Autodesk Inventor part; units mm, degrees
ref_plane "YZ Plane" through (0, 0, 0) normal (1, 0, 0) x (0, 1, 0)
ref_plane "XZ Plane" through (0, 0, 0) normal (0, 1, 0) x (-1, 0, 0)
ref_plane "XY Plane" through (0, 0, 0) normal (0, 0, 1) x (1, 0, 0)
sketch "Sketch1" plane through (0, 0, 0) normal (0, 1, 0) x (-1, 0, 0)
  line L0 (33.5, 64.5) -> (-33.5, 64.5)
  line L1 (-33.5, 64.5) -> (-33.5, -64.5)
  line L2 (-33.5, -64.5) -> (33.5, -64.5)
  line L3 (33.5, -64.5) -> (33.5, 64.5)
  line L4 (33.5, 64.5) -> (-33.5, -64.5) construction
  line L5 (-33.5, 64.5) -> (33.5, -64.5) construction
  point P0 (0, 0)
  dimension "d0" = 67
  dimension "d1" = 129
extrude "Extrusion1" add sketch "Sketch1" along normal blind 41
sketch "Sketch2" plane through (-33.5, 0, 64.5) normal (0, 0, 1) x (1, 0, 0)
  circle A0 centre (33.5, 20.5) radius 20.5
  circle A1 centre (33.5, 20.5) radius 18
  point P0 (33.5, 0)
  dimension "d4" = 41
  dimension "d5" = 36
extrude "Extrusion2" add sketch "Sketch2" along normal blind 54 contours A1
extrude "Extrusion3" add sketch "Sketch2" along normal blind 15
sketch "Sketch4" plane through (33.5, 0, -64.5) normal (0, 0, -1) x (-1, 0, 0)
  circle A0 centre (42, 20.5) radius 12.5
  line L0 (67, 0) -> (67, 41)
  point P0 (33.5, 0)
  dimension "d13" = 25
  dimension "d14" = 25
extrude "Extrusion5" add sketch "Sketch4" along normal blind 80
sketch "Sketch5" plane through (0, 0, 0) normal (0, -1, 0) x (1, 0, 0)
  circle A0 centre (0, 51.5) radius 2.5
  circle A1 centre (0, 8.5) radius 2.5
  circle A2 centre (0, -21.5) radius 2
  circle A3 centre (0, -33.5) radius 2.5
  line L0 (-2, 39.5) -> (-2, 37.5)
  line L1 (2, 37.5) -> (2, 39.5)
  arc A4 (2, 39.5) -> (-2, 39.5) centre (0, 39.5) ccw
  arc A5 (-2, 37.5) -> (2, 37.5) centre (0, 37.5) ccw
  line L2 (18, 118.5) -> (-18, 118.5)
  point P0 (2, 38.5)
  point P1 (-2, 38.5)
  dimension "d17" = 5
  dimension "d19" = 4
  dimension "d20" = 5
  dimension "d23" = 67
  dimension "d24" = 80
  dimension "d25" = 110
  dimension "d35" = 85
  dimension "d36" = 60
hole "Hole1" at (0, 0, 51.5) at (0, 0, -33.5) direction (0, 1, 0) diameter 4.917 depth 10
hole "Hole2" at (0, 0, 8.5) direction (0, 1, 0) diameter 4.9784 depth 10
hole "Hole3" at (0, 0, 39.5) at (0, 0, 37.5) at (0, 0, -21.5) direction (0, 1, 0) diameter 4 depth 10
properties part number "Updated Laser Scanner"
For this review, take the finished solid that the model builds, in its own axes (mm). A direction names the side the tool comes from. Coordinates: 2 decimals unless noted, no trailing zeros. Write each loop counter-clockwise with the first axis right and the second up, starting at its lowest first coordinate (ties: lowest second). Pieces come first, ordered by that corner, then holes.
(1) Tool access review of faces 5 (the face through (0, 10, 9)), 6 (the face through (-4.444, 40.513, 71.895)), 7 (the face through (24, 20, 64.5)): name each direction out of +Z, -Z, +X, -X, +Y, -Y from which nothing blocks a thin tool from reaching the whole face with its end or side.
(2) Add section B-B on y = 13. Give the boundary of the cut face in (x, z), then the cut area to 3 significant figures.
(3) Add section C-C on x = -8.5. Give the boundary of the cut face in (y, z), then the cut area to 3 significant figures.
(4) The part is to be moulded in two halves that separate along Z. For faces 1 (the face through (-8, 21, -144.5)), 2 (the face through (0, 10, 52)), 3 (the face through (0, 41, 1)), 4 (the face through (0.94, 5.07, -35.77)), say which applies: +Z half, -Z half, draft (parallel to the pull), parting line (faces both ways), or undercut.
(5) Wall thickness on probe 1 along Z at (x, y) = (0, 3); probe 2 along Z at (x, y) = (0, 2); probe 3 along X at (y, z) = (5.5, 8.5): over which ranges is each line inside the solid? List them lowest first.
(6) Add section A-A on z = 8.5. Give the boundary of the cut face in (x, y), then the cut area to 3 significant figures.
(7) Add section D-D on z = 51.5. Give the boundary of the cut face in (x, y).
(8) For pin 1 Ø2.5 at (x, z) = (0.5, -33.5) entering from -Y; pin 2 Ø1.5 at (y, z) = (25.5, -65.5) entering from -X; pin 3 Ø2 at (x, y) = (26, 4.5) entering from +Z, all flat-tipped, find the tip position at first contact; note any pin that passes through.
Answer sheet:
1. face 5: -Y
1. face 6: +Z
1. face 7: +Z, +X
2. outline: (-33.5, -64.5) - (-18.5, -64.5) - (-18.5, -144.5) - (1.5, -144.5) - (1.5, -64.5) - (33.5, -64.5) - (33.5, 64.5) - (19.08, 64.5) - (19.08, 79.5) - (16.36, 79.5) - (16.36, 118.5) - (-16.36, 118.5) - (-16.36, 79.5) - (-19.08, 79.5) - (-19.08, 64.5) - (-33.5, 64.5) - close
2. area: 12,100 mm2
3. outline: (0, -64.5) - (8, -64.5) - (8, -144.5) - (33, -144.5) - (33, -64.5) - (41, -64.5) - (41, 64.5) - (39.15, 64.5) - (39.15, 79.5) - (36.37, 79.5) - (36.37, 118.5) - (4.63, 118.5) - (4.63, 79.5) - (1.85, 79.5) - (1.85, 64.5) - (0, 64.5) - close
3. area: 9,090 mm2
4. face 1: -Z half
4. face 2: undercut
4. face 3: draft
4. face 4: undercut
5. probe 1: z = -64.5 to -35.96, -31.04 to -23.5, -19.5 to 6.01, 10.99 to 35.5, 41.5 to 49.04, 53.96 to 118.5
5. probe 2: z = -64.5 to -35.96, -31.04 to -23.5, -19.5 to 6.01, 10.99 to 35.5, 41.5 to 49.04, 53.96 to 79.5
5. probe 3: x = -33.5 to -2.49, 2.49 to 33.5
6. outline: (-33.5, 0) - (-2.49, 0) - (-2.49, 10) - (2.49, 10) - (2.49, 0) - (33.5, 0) - (33.5, 41) - (-33.5, 41) - close
6. area: 2,700 mm2
7. outline: (-33.5, 0) - (-2.46, 0) - (-2.46, 10) - (2.46, 10) - (2.46, 0) - (33.5, 0) - (33.5, 41) - (-33.5, 41) - close
8. pin 1: stops at y = 10
8. pin 2: stops at x = -20.26
8. pin 3: stops at z = 64.5
